from build123d import *

# Parameters (mm, degrees)
SKETCH1_R           = 12.7
BOSS_EXTRUDE1_DEPTH = 3
CHAMFER1_SIZE       = 5


with BuildPart() as part:
    # Sketch1 → Boss-Extrude1 (new body)
    with BuildSketch(Plane.XY):
        Polygon((-78.698002714, 24.844630316), (-78.698002714, 40.844630316), (-59.698002714, 40.844630316), (-8.698002714, 40.844630316), (-8.698002714, 8.844630316), (-59.698002714, 8.844630316), (-78.698002714, 8.844630316), align=None)
        with Locations((-59.698002714, 24.844630316)):
            Circle(SKETCH1_R, mode=Mode.SUBTRACT)
        with Locations((-27.698002714, 24.844630316)):
            Circle(SKETCH1_R, mode=Mode.SUBTRACT)
    extrude(amount=BOSS_EXTRUDE1_DEPTH)

    # Chamfer1
    chamfer1_edges = [part.edges().sort_by_distance(p)[0] for p in [
        (-8.698002714, 40.844630316, 1.5),
        (-78.698002714, 40.844630316, 1.5),
    ]]
    chamfer(chamfer1_edges, length=CHAMFER1_SIZE)


solid = part.part
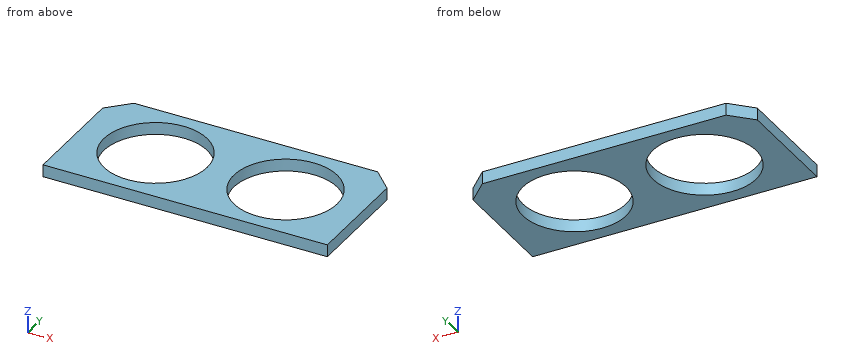
Verification items for the finished model (mm, model axes). Coordinates: 2 decimals unless noted, no trailing zeros. Order: outer loops, then holes, each group sorted by start corner. A loop starts at its lowest first (then second) coordinate and runs counter-clockwise, first axis right, second up. Notation, with made-up numbers: (21.25, 43.5) -> (56.25, 43.5) arc R24 ccw to (56.25, 64.5) -> close; hole circle Ø8 at (74.25, 70.5). An arc over 180 degrees is marked (long way). Use CSV: the item, a comma, the result in double quotes. Start each with the question number.
Q1. Thickness scan on line 1 along X through (y, z) = (21, 0.7); line 2 along X through (y, z) = (28, 0.75); line 3 along Y through (x, z) = (-35, 0.3). Record the ranges inside material, lowest first.
Q2. Section check D-D, the plane y = 29. Record the cut outline in (x, z).
Q3. Section check C-C, the plane z = 1.5. Record the cut outline in (x, y), and give its area (3 significant figures).
Q4. Section check A-A, the plane x = -58.5. Record the cut outline in (y, z), and give its area (3 significant figures).
Q5. Section check B-B, the plane y = 32.5. Record the cut outline in (x, z), and give its area (3 significant figures).
Returned:
1,line 1,"x = -78.7 to -71.8, -47.59 to -39.8, -15.59 to -8.7"
1,line 2,"x = -78.7 to -72, -47.4 to -40, -15.4 to -8.7"
1,line 3,"y = 8.84 to 14.45, 35.24 to 40.84"
2,outline,"(-78.7, 0) -> (-71.7, 0) -> (-71.7, 3) -> (-78.7, 3) -> close; (-47.7, 0) -> (-39.7, 0) -> (-39.7, 3) -> (-47.7, 3) -> close; (-15.7, 0) -> (-8.7, 0) -> (-8.7, 3) -> (-15.7, 3) -> close"
3,outline,"(-78.7, 8.84) -> (-8.7, 8.84) -> (-8.7, 35.84) -> (-13.7, 40.84) -> (-73.7, 40.84) -> (-78.7, 35.84) -> close; hole circle Ø25.4 at (-59.7, 24.84); hole circle Ø25.4 at (-27.7, 24.84)"
3,area,"1,200 mm^2"
4,outline,"(8.84, 0) -> (12.2, 0) -> (12.2, 3) -> (8.84, 3) -> close; (37.49, 0) -> (40.84, 0) -> (40.84, 3) -> (37.49, 3) -> close"
4,area,"20.1 mm^2"
5,outline,"(-78.7, 0) -> (-69.83, 0) -> (-69.83, 3) -> (-78.7, 3) -> close; (-49.56, 0) -> (-37.83, 0) -> (-37.83, 3) -> (-49.56, 3) -> close; (-17.56, 0) -> (-8.7, 0) -> (-8.7, 3) -> (-17.56, 3) -> close"
5,area,"88.4 mm^2"
